Model file for the job. Use its own axes, mm. A direction names the side the tool comes from. Coordinates: 2 decimals unless noted, no trailing zeros. Loops run counter-clockwise (first coordinate to the right, second up) from the corner with the lowest first, then second, coordinate; pieces in that order, holes last. Notation, with made-up numbers: M 82.25,23 L 90.25,23 A14 cw 90.25,33 Z; hole C 45.5,-5.75 d6. An arc over 180 degrees is marked long. One line per question, with ' | ' between items. Start each with the question number.
```python
from build123d import *

# Parameters (mm, degrees)
SKETCH1_W           = 355.6
SKETCH1_H           = 254
BOSS_EXTRUDE1_DEPTH = 36.5125
SHELL1_T            = -25.4
SKETCH2_R           = 12.7
CUT_EXTRUDE1_DEPTH  = 190.5


with BuildPart() as part:
    # Sketch1 → Boss-Extrude1 (new body, symmetric)
    with BuildSketch(Plane.XY):
        Rectangle(SKETCH1_W, SKETCH1_H)
    extrude(amount=BOSS_EXTRUDE1_DEPTH, both=True)

    # Shell1
    shell1_openings = [part.faces().sort_by_distance(p)[0] for p in [
        (0, 0, 36.5125),
    ]]
    offset(amount=SHELL1_T, openings=shell1_openings, kind=Kind.INTERSECTION)

    # Sketch2 → Cut-Extrude1 (cut)
    with BuildSketch(Plane.ZY.offset(177.8)):
        with Locations((-11.1125, 0)):
            Circle(SKETCH2_R)
    extrude(amount=-CUT_EXTRUDE1_DEPTH, mode=Mode.SUBTRACT)


solid = part.part
```
(1) Pin check, flat tips, straight feed: P1, Ø10, axis at x = 9.5, y = -89, coming from the +Z side; P2, Ø4, axis at y = 6, z = -16.5, coming from the -X side. Stop position of each tip, or through.
(2) Band-saw the part on C-C on y = 36.5. Write the cut outline in (x, z), then the cut area to 3 significant figures.
(3) Band-saw the part on A-A on z = 12.5. Write the cut outline in (x, y).
(4) Band-saw the part on D-D on x = -135.5. Write the cut outline in (y, z), then the cut area to 3 significant figures.
(5) 3-axis set-ups, long thin cutter, end or side, ignore diameter. For faces 1 (the face through (-83.9, 0.6, -23.8)), 2 (the face through (-152.4, -1, 13)), 3 (the face through (-2, 127, 1)): which of +Z, -Z, +X, -X, +Y, -Y reach the whole face in a straight line?
(6) Band-saw the part on B-B on y = 0. Write the cut outline in (x, z), then the cut area to 3 significant figures.
(7) Two-plate mould, pull along X, no slides. Class faces 4 (the face through (-2, 2, -36.512)), 5 (the face through (12.7, 0, -16)), 6 (the face through (177.8, -2, 1)), 7 (the face through (152.4, -1, 13)): pulls with the +X half, pulls with the -X half, needs draft (parallel to the pull), parting line crosses it, or undercut.
(8) Drill centre lines: line 1 (Y direction, x = 11, z = 14); line 2 (X direction, y = -90.5, z = 1.5); line 3 (Y direction, x = 12.5, z = -22.5). Where is each one in solid material? Low to high. Write a range as [from, to].
Computed values:
1) P1: z = -11.11 | P2: x = 12.7
2) outline: M -177.8,-36.51 L 177.8,-36.51 L 177.8,36.51 L 152.4,36.51 L 152.4,-11.11 L -152.4,-11.11 L -152.4,36.51 L -177.8,36.51 Z | area: 11,500 mm^2
3) outline: M -177.8,-127 L 177.8,-127 L 177.8,127 L -177.8,127 Z; hole M -152.4,-101.6 L 152.4,-101.6 L 152.4,101.6 L -152.4,101.6 Z
4) outline: M -127,-36.51 L 127,-36.51 L 127,36.51 L 101.6,36.51 L 101.6,-11.11 L 12.7,-11.11 A12.7 cw -12.7,-11.11 L -101.6,-11.11 L -101.6,36.51 L -127,36.51 Z | area: 8,620 mm^2
5) face 1: -X | face 2: +Z | face 3: +Z, -Z, +X, -X, +Y
6) outline: M -177.8,-36.51 L 177.8,-36.51 L 177.8,36.51 L 152.4,36.51 L 152.4,-11.11 L 12.7,-11.11 L 12.7,-23.81 L -177.8,-23.81 Z; M -177.8,1.59 L -152.4,1.59 L -152.4,36.51 L -177.8,36.51 Z | area: 8,710 mm^2
7) face 4: needs draft | face 5: pulls with the -X half | face 6: pulls with the +X half | face 7: undercut
8) line 1: [-127, -101.6], [101.6, 127] | line 2: [-177.8, -152.4], [152.4, 177.8] | line 3: [-127, -5.62], [5.62, 127]
